Drawing for the job (mm, zero at the part's lowest x, y, z). Give positions to 0.01 mm unless a question says otherwise; leave off trailing zeros. Order: outer loops, then holes, each group sorted by start corner. A loop starts at its lowest first (then second) coordinate and runs counter-clockwise, first axis right, second up. Notation, with made-up numbers: (79.25, 40) -> (117.25, 40) arc R31 cw to (117.25, 68) -> close; hole circle Ø2 at (-19, 18). An arc over 180 degrees is marked (long way). Use one line per item in the form item = value. Start each with the question number.
1) Mould opens along Y. For the marked faces 1, 2 and 3 say: pulls with the +Y half, pulls with the -Y half, needs draft (parallel to the pull), parting line crosses it, or undercut.
2) Cut at A-A, the plane z = 5. Give the cut face in (x, y).
3) Probe line 1 (X direction, y = 2.05, z = 3.25) (1 decimal); line 2 (Y direction, x = 2.05, z = 3.5); line 3 (X direction, y = 3.55, z = 5.25) (1 decimal). List the from-to ranges inside material, lowest first.
4) Cut at C-C, the plane x = 3.2. Give the cut face in (y, z).
5) Cut at D-D, the plane x = 0.75. Give the cut face in (y, z).
6) Cut at B-B, the plane y = 1.5. Give the cut face in (x, z).
7) Drop flat-ended pins along their axis: P1, Ø1, axis at x = 5, z = 11.5, coming from the -Y side (1 decimal); P2, Ø1, axis at y = 4.5, z = 13.5, coming from the -X side (1 decimal); P3, Ø1, axis at y = 1, z = 12, coming from the +X side; P4, Ø3, axis at x = 2.89, y = 2.5, coming from the +Z side. Give the stop position or say it passes through.
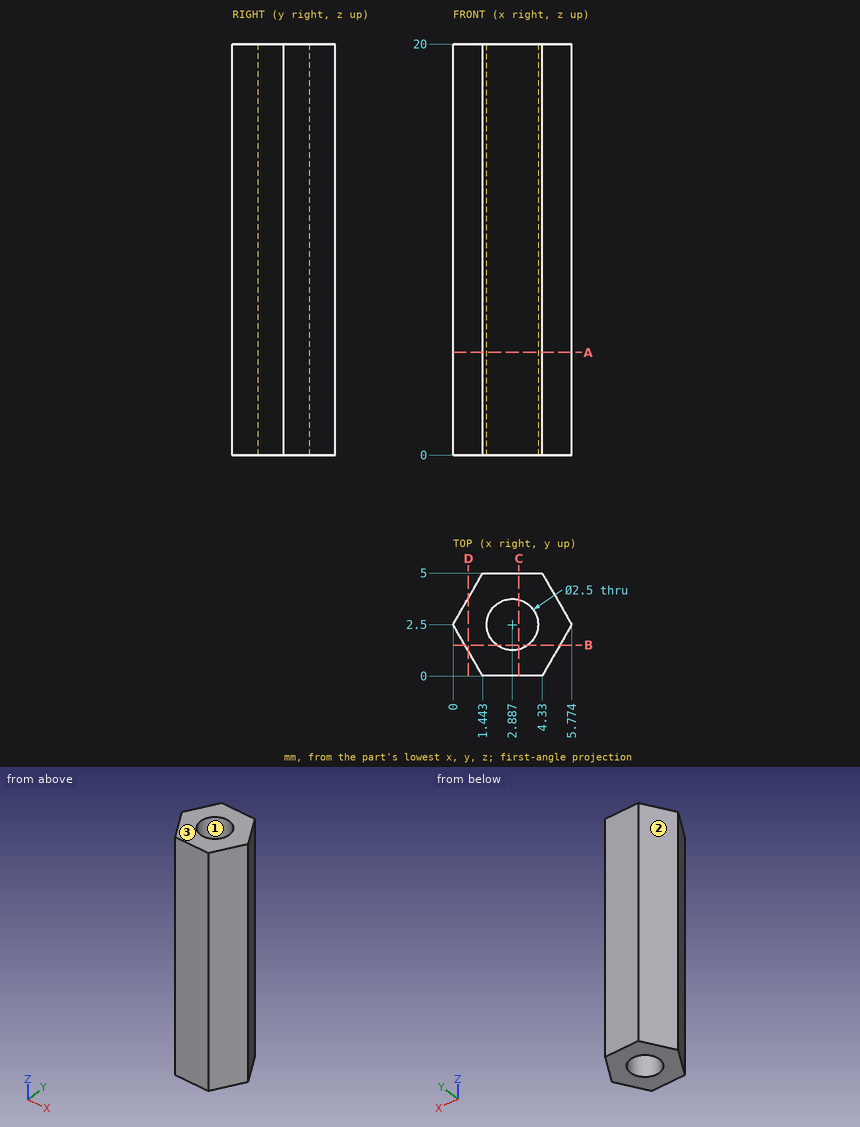
Result:
q1.face_1 = undercut
q1.face_2 = pulls with the +Y half
q1.face_3 = needs draft
q2.outline = (0, 2.5) -> (1.44, 0) -> (4.33, 0) -> (5.77, 2.5) -> (4.33, 5) -> (1.44, 5) -> close; hole circle Ø2.5 at (2.89, 2.5)
q3.line_1 = 0.3 to 1.7, 4.1 to 5.5
q3.line_2 = 0 to 1.57, 3.43 to 5
q3.line_3 = 0.6 to 2.2, 3.6 to 5.2
q4.outline = (0, 0) -> (1.29, 0) -> (1.29, 20) -> (0, 20) -> close; (3.71, 0) -> (5, 0) -> (5, 20) -> (3.71, 20) -> close
q5.outline = (1.2, 0) -> (3.8, 0) -> (3.8, 20) -> (1.2, 20) -> close
q6.outline = (0.58, 0) -> (2.14, 0) -> (2.14, 20) -> (0.58, 20) -> close; (3.64, 0) -> (5.2, 0) -> (5.2, 20) -> (3.64, 20) -> close
q7.P1 = 0.3
q7.P2 = 0.9
q7.P3 = 5.2
q7.P4 = 20
